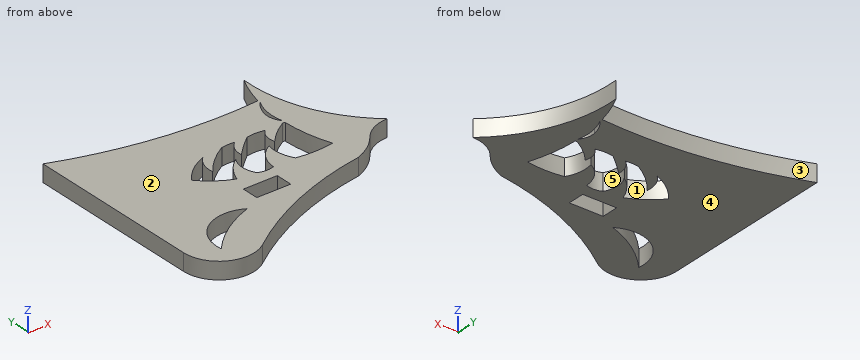
from build123d import *

# Parameters (mm, degrees)
SKETCH1_W           = 3.048
SKETCH1_H           = 1.524
BOSS_EXTRUDE1_DEPTH = 1.524
FILLET4_R           = 3.175


with BuildPart() as part:
    # Sketch1 → Boss-Extrude1 (new body)
    with BuildSketch(Plane.XY):
        with BuildLine():
            Line((0.680153889, -6.129418594), (0.680153889, 11.540681963))
            ThreePointArc((0.680153889, 11.540681963), (9.222616512, 9.36144264), (18.034529819, 9.091376803))
            ThreePointArc((18.034529819, 9.091376803), (18.476514137, 10.575327988), (19.079546917, 12.001446047))
            ThreePointArc((19.079546917, 12.001446047), (20.097392283, 6.202497031), (23.594187572, 1.465806036))
            ThreePointArc((23.594187572, 1.465806036), (22.264781917, 1.159048918), (21.169318906, 0.345796118))
            ThreePointArc((21.169318906, 0.345796118), (20.057462236, -0.769306292), (18.675392755, -1.524))
            ThreePointArc((18.675392755, -1.524), (10.681603645, -3.986495409), (3.71145902, -8.610523078))
            ThreePointArc((3.71145902, -8.610523078), (1.563251963, -8.142798296), (0.680153889, -6.129418594))
        make_face()
        with Locations((11.054430571, -0.762)):
            Rectangle(SKETCH1_W, SKETCH1_H, mode=Mode.SUBTRACT)
        with BuildLine():
            ThreePointArc((18.457205049, 1.159048918), (16.796602855, 1.012131062), (15.13600066, 1.159048918))
            ThreePointArc((15.13600066, 1.159048918), (14.678205729, 2.355037825), (14.715312916, 3.635111542))
            ThreePointArc((14.715312916, 3.635111542), (13.593992305, 2.610148755), (13.144305869, 1.159048918))
            ThreePointArc((13.144305869, 1.159048918), (12.426226698, 1.043141082), (11.720524566, 1.219370545))
            ThreePointArc((11.720524566, 1.219370545), (11.364676413, 2.427241044), (11.720524566, 3.635111542))
            ThreePointArc((11.720524566, 3.635111542), (10.712351561, 2.650528395), (10.061249405, 1.400775314))
            ThreePointArc((10.061249405, 1.400775314), (8.64082558, 2.160669947), (7.450155331, 3.245726654))
            ThreePointArc((7.450155331, 3.245726654), (8.601081625, 4.454929507), (10.061249405, 5.264072837))
            ThreePointArc((10.061249405, 5.264072837), (9.457771061, 4.34236946), (9.352425063, 3.245726654))
            ThreePointArc((9.352425063, 3.245726654), (10.543430802, 4.522443251), (11.971709271, 5.526694491))
            ThreePointArc((11.971709271, 5.526694491), (12.557411502, 5.573473862), (13.144305869, 5.545359518))
            ThreePointArc((13.144305869, 5.545359518), (12.566006589, 4.808091463), (12.426226698, 3.881562551))
            ThreePointArc((12.426226698, 3.881562551), (13.312490945, 4.743692313), (14.253799466, 5.545359518))
            ThreePointArc((14.253799466, 5.545359518), (15.051720121, 5.625849498), (15.84620994, 5.516570329))
            ThreePointArc((15.84620994, 5.516570329), (15.396051863, 4.760868409), (15.419480332, 3.881562551))
            ThreePointArc((15.419480332, 3.881562551), (16.340692115, 4.785475695), (17.404266633, 5.516570329))
            ThreePointArc((17.404266633, 5.516570329), (17.532648387, 5.563352566), (17.656087794, 5.504759346))
            ThreePointArc((17.656087794, 5.504759346), (17.884238381, 3.300121283), (18.457205049, 1.159048918))
        make_face(mode=Mode.SUBTRACT)
        with BuildLine():
            ThreePointArc((17.656087794, 5.840129035), (17.574660077, 7.375234106), (18.034529819, 8.84210079))
            ThreePointArc((18.034529819, 8.84210079), (17.521152532, 8.084430816), (17.246705878, 7.211333419))
            ThreePointArc((17.246705878, 7.211333419), (17.311898149, 6.484082994), (17.656087794, 5.840129035))
        make_face(mode=Mode.SUBTRACT)
        with BuildLine():
            ThreePointArc((8.037489597, -2.327562697), (5.34711842, -3.636841183), (3.096001374, -5.607825523))
            ThreePointArc((3.096001374, -5.607825523), (4.535873462, -2.414756972), (8.037489597, -2.327562697))
        make_face(mode=Mode.SUBTRACT)
    extrude(amount=BOSS_EXTRUDE1_DEPTH)

    # Fillet4
    fillet4_edges = [part.edges().sort_by_distance(p)[0] for p in [
        (3.71145902, -8.610523078, 0.762),
    ]]
    fillet(fillet4_edges, radius=FILLET4_R)


solid = part.part
Verification items for the finished model (mm, model axes). Face numbers are marked on the shaded views. A direction names the side the tool comes from. Coordinates: 2 decimals unless noted, no trailing zeros. Order: outer loops, then holes, each group sorted by start corner. A loop starts at its lowest first (then second) coordinate and runs counter-clockwise, first axis right, second up.
Item 1: Section check D-D, the plane y = -0.75. Enter the section's corners in (x, z), then the cut area to 3 significant figures.
Filled in:
outline: (0.68, 0) - (9.53, 0) - (9.53, 1.52) - (0.68, 1.52) - close; (12.58, 0) - (20.08, 0) - (20.08, 1.52) - (12.58, 1.52) - close
area: 24.9 mm2
Item 2: Release check for a two-part mould opening along Y. For the marked faces 1, 2 and 3 record: +Y half, -Y half, draft (parallel to the pull), parting line (faces both ways), or undercut.
Filled in:
face 1: undercut
face 2: draft
face 3: +Y half
Item 3: Access from +Z, -Z, +X, -X, +Y, -Y to the whole of each face (thin tool, end or side, straight path). Record for the marked faces 4 and 5.
Filled in:
face 4: -Z, +X, -X, +Y, -Y
face 5: +Z, -Z
Item 4: Section check B-B, the plane y = 2.75. Enter the section's corners in (x, z).
Filled in:
outline: (0.68, 0) - (7.92, 0) - (7.92, 1.52) - (0.68, 1.52) - close; (10.79, 0) - (11.39, 0) - (11.39, 1.52) - (10.79, 1.52) - close; (13.69, 0) - (14.64, 0) - (14.64, 1.52) - (13.69, 1.52) - close; (18, 0) - (22.28, 0) - (22.28, 1.52) - (18, 1.52) - close
Item 5: Material ranges on L1, parallel to Y at x = 17.5, z = 0.8; L2, parallel to X at y = 2.5, z = 1.3; L3, parallel to X at y = 4.5, z = 1.15, recorded low to high.
Filled in:
L1: y = -1.73 to 1.04, 5.56 to 6.06, 8.04 to 9.05
L2: x = 0.68 to 8.2, 10.61 to 11.37, 13.53 to 14.66, 18.06 to 22.51
L3: x = 0.68 to 8.66, 9.52 to 10.52, 12.46 to 13.05, 15.35 to 16.01, 17.72 to 20.98
Item 6: Section check C-C, the plane z = 0.45. Give the number of separate pieces and of enclosed holes in the cut face, then the cut area to 3 significant figures.
Filled in:
separate pieces: 1
enclosed holes: 4
area: 238 mm2
Item 7: Section check A-A, the plane y = 8.25. Enter the section's corners in (x, z).
Filled in:
outline: (0.68, 0) - (17.61, 0) - (17.61, 1.52) - (0.68, 1.52) - close; (17.78, 0) - (19.42, 0) - (19.42, 1.52) - (17.78, 1.52) - close
